```python
from build123d import *

# Parameters (mm, degrees)
BASE_EXTRUDE_DEPTH   = 2.5
FILLET1_R            = 4
BOSS_EXTRUDE1_DEPTH  = 1.5
FILLET2_R            = 0.75
SKETCH4_R            = 4
BOSS_EXTRUDE2_DEPTH  = 0.25
SKETCH5_R            = 3.475
BOSS_EXTRUDE7_DEPTH  = 2
CUT_EXTRUDE2_DEPTH   = 129.647930415
FILLET2_OF_MIRROR1_R = 0.75
BOSS_EXTRUDE8_DEPTH  = 0.75
FILLET3_R            = 0.75
SKETCH8_R            = 9.25
SKETCH8_R_2          = 8
BOSS_EXTRUDE9_DEPTH  = 1.8
SKETCH9_W            = 2
SKETCH9_H            = 27.383801512
CUT_EXTRUDE3_DEPTH   = 0.5
LPATTERN1_COUNT      = 6
LPATTERN1_PITCH      = 4
SKETCH10_W           = 2
SKETCH10_H           = 27.383801512
CUT_EXTRUDE4_DEPTH   = 0.5
LPATTERN2_COUNT      = 4
LPATTERN2_PITCH      = 4


# Some blends are built 0.0001 mm under size
with BuildPart() as part:
    # Sketch1 → Base-Extrude (new body)
    with BuildSketch(Plane(origin=(0, 0, 0), x_dir=(1, 0, 0), z_dir=(0, 1, 0))):
        with BuildLine():
            Line((4, 0), (118, 0))
            ThreePointArc((118, 0), (121.535533906, 1.464466094), (123, 5))
            Line((123, 5), (123, 29.8))
            ThreePointArc((123, 29.8), (121.535533906, 33.335533906), (118, 34.8))
            Line((118, 34.8), (4, 34.8))
            ThreePointArc((4, 34.8), (1.171572875, 33.628427125), (0, 30.8))
            Line((0, 30.8), (0, 4))
            ThreePointArc((0, 4), (1.171572875, 1.171572875), (4, 0))
        make_face()
    extrude(amount=BASE_EXTRUDE_DEPTH)

    # Fillet1
    # the kernel refuses this fillet: 4 mm, written as the material it takes off along each edge
    with BuildSketch(Plane(origin=(118, 2.5, -5), x_dir=(0, 0, 1), z_dir=(-1, 0, 0))) as fillet1_piece_1:
        with BuildLine():
            CenterArc((1.291900756, -4), FILLET1_R, 22.024312837, 67.975687163)
            Line((1.291900756, 0), (1.291900756, 0.08))
            Line((1.291900756, 0.08), (5, 0.08))
            Line((5, 0.08), (5.08, 0))
            ThreePointArc((5.08, 0), (5.08, -1.25), (5.074161985, -2.47))
            Line((5.074161985, -2.47), (5, -2.5))
        make_face()
    revolve(axis=Axis((118, 2.5, -5), (0, 1, 0)), revolution_arc=90, mode=Mode.SUBTRACT)
    with BuildSketch(Plane(origin=(123, 2.5, -5), x_dir=(0, -1, 0), z_dir=(0, 0, -1))) as fillet1_piece_2:
        with BuildLine():
            CenterArc((4, 3.708099244), FILLET1_R, 180, 67.975687163)
            Line((0, 3.708099244), (-0.08, 3.708099244))
            Line((-0.08, 3.708099244), (-0.08, 0))
            Line((-0.08, 0), (0, -0.08))
            ThreePointArc((0, -0.08), (1.25, -0.08), (2.47, -0.074161985))
            Line((2.47, -0.074161985), (2.5, 0))
        make_face()
    extrude(amount=24.8, mode=Mode.SUBTRACT)
    with BuildSketch(Plane(origin=(118, 2.5, -29.8), x_dir=(1, 0, 0), z_dir=(0, 0, 1))) as fillet1_piece_3:
        with BuildLine():
            CenterArc((1.291900756, -4), FILLET1_R, 22.024312837, 67.975687163)
            Line((1.291900756, 0), (1.291900756, 0.08))
            Line((1.291900756, 0.08), (5, 0.08))
            Line((5, 0.08), (5.08, 0))
            ThreePointArc((5.08, 0), (5.08, -1.25), (5.074161985, -2.47))
            Line((5.074161985, -2.47), (5, -2.5))
        make_face()
    revolve(axis=Axis((118, 2.5, -29.8), (0, 1, 0)), revolution_arc=90, mode=Mode.SUBTRACT)
    with BuildSketch(Plane(origin=(118, 2.5, -34.8), x_dir=(0, -1, 0), z_dir=(-1, 0, 0)), Plane(origin=(4, 2.5, 0), x_dir=(0, -1, 0), z_dir=(1, 0, 0))) as fillet1_piece_4:
        with BuildLine():
            CenterArc((4, 3.708099244), FILLET1_R, 180, 67.975687163)
            Line((0, 3.708099244), (-0.08, 3.708099244))
            Line((-0.08, 3.708099244), (-0.08, 0))
            Line((-0.08, 0), (0, -0.08))
            ThreePointArc((0, -0.08), (1.25, -0.08), (2.47, -0.074161985))
            Line((2.47, -0.074161985), (2.5, 0))
        make_face()
    extrude(amount=114, mode=Mode.SUBTRACT)
    with BuildSketch(Plane(origin=(4, 2.5, -30.8), x_dir=(0, 0, -1), z_dir=(1, 0, 0))) as fillet1_piece_5:
        with BuildLine():
            CenterArc((0.291900756, -4), FILLET1_R, 22.024312837, 67.975687163)
            Line((0.291900756, 0), (0.291900756, 0.08))
            Line((0.291900756, 0.08), (4, 0.08))
            Line((4, 0.08), (4.08, 0))
            ThreePointArc((4.08, 0), (4.08, -1.25), (4.074161985, -2.47))
            Line((4.074161985, -2.47), (4, -2.5))
        make_face()
    revolve(axis=Axis((4, 2.5, -30.8), (0, 1, 0)), revolution_arc=90, mode=Mode.SUBTRACT)
    with BuildSketch(Plane(origin=(0, 2.5, -30.8), x_dir=(0, -1, 0), z_dir=(0, 0, 1))) as fillet1_piece_6:
        with BuildLine():
            CenterArc((4, 3.708099244), FILLET1_R, 180, 67.975687163)
            Line((0, 3.708099244), (-0.08, 3.708099244))
            Line((-0.08, 3.708099244), (-0.08, 0))
            Line((-0.08, 0), (0, -0.08))
            ThreePointArc((0, -0.08), (1.25, -0.08), (2.47, -0.074161985))
            Line((2.47, -0.074161985), (2.5, 0))
        make_face()
    extrude(amount=26.8, mode=Mode.SUBTRACT)
    with BuildSketch(Plane(origin=(4, 2.5, -4), x_dir=(-1, 0, 0), z_dir=(0, 0, -1))) as fillet1_piece_7:
        with BuildLine():
            CenterArc((0.291900756, -4), FILLET1_R, 22.024312837, 67.975687163)
            Line((0.291900756, 0), (0.291900756, 0.08))
            Line((0.291900756, 0.08), (4, 0.08))
            Line((4, 0.08), (4.08, 0))
            ThreePointArc((4.08, 0), (4.08, -1.25), (4.074161985, -2.47))
            Line((4.074161985, -2.47), (4, -2.5))
        make_face()
    revolve(axis=Axis((4, 2.5, -4), (0, 1, 0)), revolution_arc=90, mode=Mode.SUBTRACT)

    # Sketch3 → Boss-Extrude1 (add)
    with BuildSketch(Plane.XY.offset(-3.25)):
        with BuildLine():
            Line((5, 0), (111, 0))
            Line((111, 0), (111, -1.5))
            Line((111, -1.5), (48.5, -1.5))
            Line((48.5, -1.5), (43.075167447, -10.977404274))
            ThreePointArc((43.075167447, -10.977404274), (37, -14.5), (30.924832553, -10.977404274))
            Line((30.924832553, -10.977404274), (25.5, -1.5))
            Line((25.5, -1.5), (5, -1.5))
            Line((5, -1.5), (5, 0))
        make_face()
    boss_extrude1 = extrude(amount=-BOSS_EXTRUDE1_DEPTH)

    # Fillet2
    fillet2_edges = [part.edges().sort_by_distance(p)[0] for p in [
        (5, -0.75, -4.75),
        (111, -0.75, -3.25),
        (111, -0.75, -4.75),
        (5, -0.75, -3.25),
    ]]
    fillet(fillet2_edges, radius=FILLET2_R - 0.0001)  # a hair under: the kernel refuses the full size

    # Sketch4 → Boss-Extrude2 (add)
    with BuildSketch(Plane.XY.offset(-3.25)):
        with Locations(Location((37, -7.5, 0), (0, 0, 180))):
            Circle(SKETCH4_R)
    boss_extrude2 = extrude(amount=BOSS_EXTRUDE2_DEPTH)

    # Sketch5 → Boss-Extrude7 (add)
    with BuildSketch(Plane.XY.offset(-3.25)):
        with Locations((37, -7.5)):
            Circle(SKETCH5_R)
    boss_extrude7 = extrude(amount=BOSS_EXTRUDE7_DEPTH)

    # Sketch6 → Cut-Extrude2 (cut, through all)
    with BuildSketch(Plane(origin=(0, 0, 0), x_dir=(0, 0, -1), z_dir=(1, 0, 0))):
        Polygon((-18.452365233, 70.746536211), (1.25, -7.5), (2.125, -10.975), (21.827365233, -89.221536211), (-134.665707189, -128.626266677), (-174.945437655, 31.341805745), align=None)
    cut_extrude2 = extrude(amount=CUT_EXTRUDE2_DEPTH, mode=Mode.SUBTRACT)

    # Mirror1: Boss-Extrude1, Boss-Extrude2, Boss-Extrude7, Cut-Extrude2 across plane
    add(boss_extrude1.mirror(Plane.XY.offset(-17.4)))
    add(boss_extrude2.mirror(Plane.XY.offset(-17.4)))
    add(boss_extrude7.mirror(Plane.XY.offset(-17.4)))
    add(cut_extrude2.mirror(Plane.XY.offset(-17.4)), mode=Mode.SUBTRACT)

    # Fillet2 of Mirror1
    fillet2_of_mirror1_edges = [part.edges().sort_by_distance(p)[0] for p in [
        (5, -0.75, -30.05),
        (111, -0.75, -31.55),
        (111, -0.75, -30.05),
        (5, -0.75, -31.55),
    ]]
    fillet(fillet2_of_mirror1_edges, radius=FILLET2_OF_MIRROR1_R - 0.0001)  # a hair under: the kernel refuses the full size

    # Sketch7 → Boss-Extrude8 (add)
    with BuildSketch(Plane.XZ):
        with BuildLine():
            Line((119.5, -30.8), (119.5, -4))
            ThreePointArc((119.5, -4), (118.75, -3.25), (118, -4))
            Line((118, -4), (118, -30.8))
            ThreePointArc((118, -30.8), (118.75, -31.55), (119.5, -30.8))
        make_face()
    extrude(amount=BOSS_EXTRUDE8_DEPTH)

    # Fillet3
    fillet3_edges = [part.edges().sort_by_distance(p)[0] for p in [
        (118.75, -0.75, -31.55),
        (118.75, -0.75, -3.25),
        (119.5, -0.75, -17.4),
        (118, -0.75, -17.4),
    ]]
    fillet(fillet3_edges, radius=FILLET3_R - 0.0001)  # a hair under: the kernel refuses the full size

    # Sketch8 → Boss-Extrude9 (add)
    with BuildSketch(Plane.XZ):
        with Locations(Location((14.5, -17.4, 0), (0, 0, 90))):
            Circle(SKETCH8_R)
        with Locations(Location((14.5, -17.4, 0), (0, 0, 270))):
            Circle(SKETCH8_R_2, mode=Mode.SUBTRACT)
    extrude(amount=BOSS_EXTRUDE9_DEPTH)

    # Sketch9 → Cut-Extrude3 (cut)
    with BuildSketch(Plane(origin=(0, 2.5, 0), x_dir=(-1, 0, 0), z_dir=(0, 1, 0))):
        with Locations((-111, -17.4)):
            Rectangle(SKETCH9_W, SKETCH9_H)
    cut_extrude3 = extrude(amount=-CUT_EXTRUDE3_DEPTH, mode=Mode.SUBTRACT)

    # LPattern1: Cut-Extrude3 ×6
    with Locations(*[(-i * LPATTERN1_PITCH, 0, 0) for i in range(1, LPATTERN1_COUNT)]):
        add(cut_extrude3, mode=Mode.SUBTRACT)

    # Sketch10 → Cut-Extrude4 (cut)
    with BuildSketch(Plane(origin=(-102, 2.5, 0), x_dir=(-1, 0, 0), z_dir=(0, 1, 0))):
        with Locations((-111, -17.4)):
            Rectangle(SKETCH10_W, SKETCH10_H)
    cut_extrude4 = extrude(amount=-CUT_EXTRUDE4_DEPTH, mode=Mode.SUBTRACT)

    # LPattern2: Cut-Extrude4 ×4
    with Locations(*[(i * LPATTERN2_PITCH, 0, 0) for i in range(1, LPATTERN2_COUNT)]):
        add(cut_extrude4, mode=Mode.SUBTRACT)


solid = part.part
```
Model file for the job. Use its own axes, mm. A direction names the side the tool comes from. Coordinates: 2 decimals unless noted, no trailing zeros. Order: outer loops, then holes, each group sorted by start corner. A loop starts at its lowest first (then second) coordinate and runs counter-clockwise, first axis right, second up. Notation, with made-up numbers: M 51,-30.75 L 98,-30.75 A9 ccw 98,-20.75 Z; hole C 81,27 d9. An arc over 180 degrees is marked long. Answer as CSV lines item,"result".
(1) 3-axis set-ups, long thin cutter, end or side, ignore diameter. For faces 1 (the flat face through (13, 2, -17)), 2 (the flat face through (37, -6, -1.25)), 3 (the flat face through (97, 2.5, -18)): which of +Z, -Z, +X, -X, +Y, -Y reach the whole face in a straight line?
Geometry says:
face 1,"+Y"
face 2,"+Z, +X, -X, -Y"
face 3,"+Z, -Z, +X, -X, +Y"
(2) Band-saw the part on B-B, the plane y = -13. List the corners of the cut face in (x, z), then the cut area to 3 significant figures.
Geometry says:
outline,"M 32.67,-31.55 L 41.33,-31.55 L 41.33,-30.05 L 32.67,-30.05 Z; M 32.67,-4.75 L 41.33,-4.75 L 41.33,-3.25 L 32.67,-3.25 Z"
area,"26.0 mm2"
(3) Wall check: line 1 along X through (y, z) = (-0.5, -17.4); line 2 along X through (y, z) = (-1.3, -17.4); line 3 along Z through (x, y) = (108, -0.5). Give the ranges that are in metal, low to high.
Geometry says:
line 1,"x = 5.25 to 6.5, 22.5 to 23.75, 118.19 to 119.31"
line 2,"x = 5.25 to 6.5, 22.5 to 23.75"
line 3,"z = -31.55 to -30.05, -4.75 to -3.25"
(4) Pull direction Z, two halves, no side cores. Call faces 4 (the flat face through (14, 0, -18)), 5 (the flat face through (19, 2.5, -18)), 6 (the cylindrical face through (60.202, 1.835, -1.5)): +Z half, -Z half, draft (parallel to the pull), parting line (faces both ways), or undercut.
Geometry says:
face 4,"undercut"
face 5,"draft"
face 6,"+Z half"
(5) Band-saw the part on A-A, the plane x = 72.5. List the corners of the cut face in (y, z), then the cut area to 3 significant figures.
Geometry says:
outline,"M -1.5,-31.55 L 0,-31.55 L 0,-34.8 A4 ccw 2.5,-31.09 L 2.5,-3.71 A4 ccw 0,0 L 0,-3.25 L -1.5,-3.25 L -1.5,-4.75 L 0,-4.75 L 0,-30.05 L -1.5,-30.05 Z"
area,"86.4 mm2"
(6) Flat gauge pins, fed straight in: pin 1 (8 mm diameter, centred on y = -1, z = -22.5, fed in from +X); pin 2 (8 mm diameter, centred on x = 13.5, z = -29, fed in from -Y); pin 3 (10 mm diameter, centred on x = 47, z = -19.5, fed in from -Y). Where does each tip first touch, or does it go through?
Geometry says:
pin 1,"stops at x = 123"
pin 2,"stops at y = -1.8"
pin 3,"stops at y = 0"
